Answer from the drawing. Dimensions are ordinates in mm from the lowest x, y and z of the part. A direction names the side the tool comes from. Coordinates: 2 decimals unless noted, no trailing zeros. Order: outer loops, then holes, each group sorted by start corner. A loop starts at its lowest first (then second) coordinate and runs counter-clockwise, first axis right, second up. Notation, with made-up numbers: (-15, 18) - (12, 18) arc R22 ccw to (12, 50) - close; hole circle Ø3 at (12.25, -16). An arc over 180 degrees is marked (long way). Use a Markdown table: item, result. Add a question column.
Item 1: For the marked faces 1 and 2, determine the directions among +Z, -Z, +X, -X, +Y, -Y from which every point of the face is accessible in a straight line to the end or side of a thin tool.
Item 2: The part is cut by section C-C, the plane y = 15.75. Give the vertices of the cut face in (x, z) (1 decimal).
Item 3: Flat-ended cylindrical pins translate along their axes: P1, Ø1.3, axis at x = 3, y = 0.5, coming from the -Z side; P2, Ø1.5, axis at y = 3, z = 0.5, coming from the +X side; P3, Ø0.8, axis at y = 0.5, z = 2.5, coming from the -X side; P4, Ø0.5, axis at y = 1, z = 2.5, coming from the +X side. Find the tip coordinate at first contact, or state that the pin passes through.
Item 4: Find the intervals of material crossed by line 1 along Y through (x, z) = (2.75, 1.65); line 2 along Z through (x, y) = (1.5, 21.5) (1 decimal); line 3 along Y through (x, z) = (0.6, 0.35), in increasing order.
Item 5: The mould has two halves that part along Y. Classify the marked faces 3, 4 and 5: released by +Y, released by -Y, zero draft, split by the parting line, or undercut.
Item 6: The part is cut by section B-B, the plane z = 0.55. Give the vertices of the cut face in (x, y).
Item 7: The part is cut by section A-A, the plane x = 3.1. Give the vertices of the cut face in (y, z) (1 decimal).
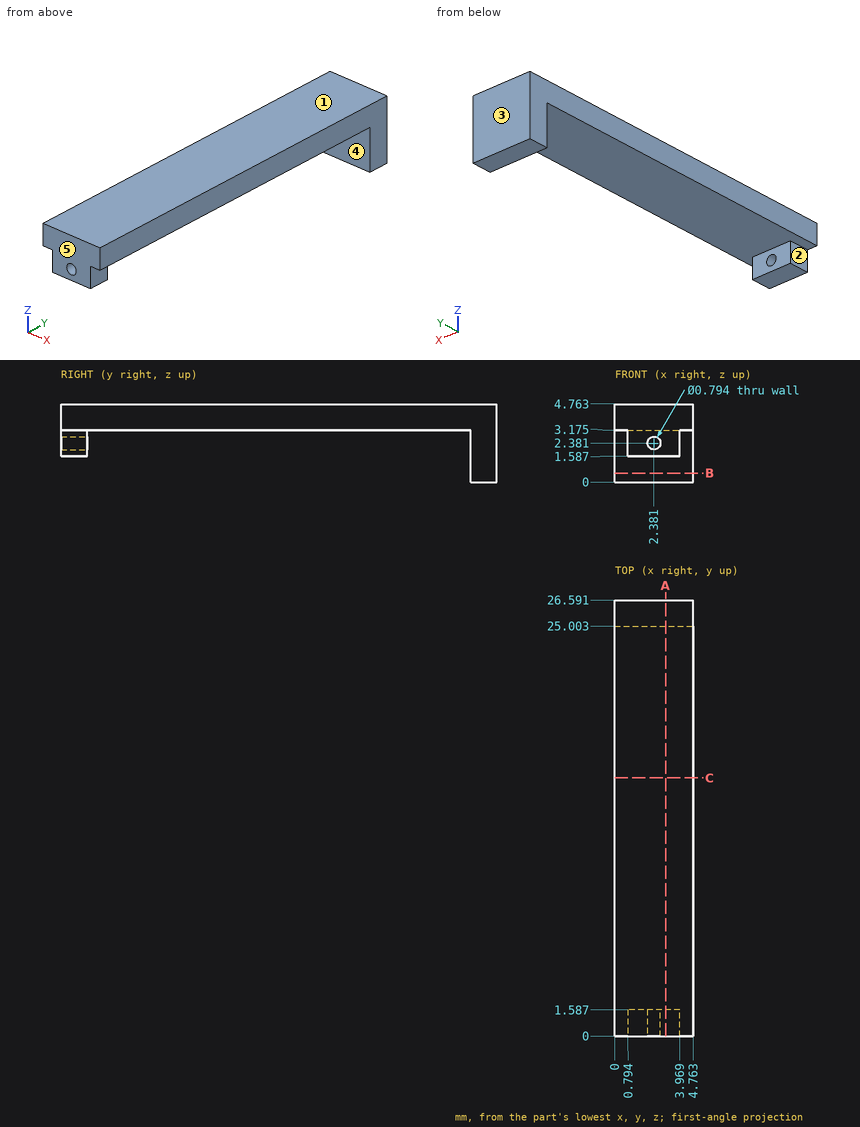
Solution:
| question | item | result |
|---|---|---|
| 1 | face 1 | +Z, +X, -X, +Y, -Y |
| 1 | face 2 | -Z, -X, -Y |
| 2 | outline | (0, 3.2) - (4.8, 3.2) - (4.8, 4.8) - (0, 4.8) - close |
| 3 | P1 | stops at z = 1.59 |
| 3 | P2 | passes through |
| 3 | P3 | stops at x = 0.79 |
| 3 | P4 | stops at x = 3.97 |
| 4 | line 1 | y = 0 to 1.59, 25 to 26.59 |
| 4 | line 2 | z = 3.2 to 4.8 |
| 4 | line 3 | y = 25 to 26.59 |
| 5 | face 3 | released by +Y |
| 5 | face 4 | undercut |
| 5 | face 5 | released by -Y |
| 6 | outline | (0, 25) - (4.76, 25) - (4.76, 26.59) - (0, 26.59) - close |
| 7 | outline | (0, 1.6) - (1.6, 1.6) - (1.6, 3.2) - (25, 3.2) - (25, 0) - (26.6, 0) - (26.6, 4.8) - (0, 4.8) - close |
